```python
from build123d import *

# Parameters (mm, degrees)
SKETCH1_W           = 76.2
SKETCH1_H           = 76.2
BOSS_EXTRUDE1_DEPTH = 2.9718
SKETCH2_W           = 2.9718
SKETCH2_H           = 38.1
CUT_EXTRUDE1_DEPTH  = 54.963428313
CUT_EXTRUDE7_DEPTH  = 54.963428313
SKETCH8_W           = 1.7526
SKETCH8_H           = 2.38125
CUT_EXTRUDE8_DEPTH  = 54.963428313


with BuildPart() as part:
    # Sketch1 → Boss-Extrude1 (new body)
    with BuildSketch(Plane(origin=(0, 0, 0), x_dir=(1, 0, 0), z_dir=(0, 1, 0))):
        Rectangle(SKETCH1_W, SKETCH1_H)
    extrude(amount=BOSS_EXTRUDE1_DEPTH)

    # Sketch2 → Cut-Extrude1 (cut, through all)
    with BuildSketch(Plane(origin=(0, 2.9718, 0), x_dir=(1, 0, 0), z_dir=(0, 1, 0))):
        with Locations((36.6141, 0)):
            Rectangle(SKETCH2_W, SKETCH2_H)
    cut_extrude1 = extrude(amount=-CUT_EXTRUDE1_DEPTH, mode=Mode.SUBTRACT)

    # Sketch7 → Cut-Extrude7 (cut, through all)
    with BuildSketch(Plane(origin=(0, 2.9718, 0), x_dir=(1, 0, 0), z_dir=(0, 1, 0))):
        Polygon((35.1282, 1.4224), (29.05125, 1.4224), (29.05125, 3.175), (26.67, 3.175), (26.67, 1.4224), (22.86, 1.4224), (22.86, -1.4224), (26.67, -1.4224), (26.67, -3.175), (29.05125, -3.175), (29.05125, -1.4224), (35.1282, -1.4224), align=None)
    cut_extrude7 = extrude(amount=-CUT_EXTRUDE7_DEPTH, mode=Mode.SUBTRACT)

    # Sketch8 → Cut-Extrude8 (cut, through all)
    with BuildSketch(Plane(origin=(0, 2.9718, 0), x_dir=(1, 0, 0), z_dir=(0, 1, 0))):
        Polygon((25.4, 38.1), (-12.7, 38.1), (-12.7, 35.1282), (4.9276, 35.1282), (7.7724, 35.1282), (25.4, 35.1282), align=None)
        Polygon((7.7724, 35.1282), (4.9276, 35.1282), (4.9276, 29.05125), (4.9276, 26.67), (4.9276, 22.86), (7.7724, 22.86), (7.7724, 26.67), (7.7724, 29.05125), align=None)
        with Locations((8.6487, 27.860625)):
            Rectangle(SKETCH8_W, SKETCH8_H)
        with Locations((4.0513, 27.860625)):
            Rectangle(SKETCH8_W, SKETCH8_H)
    extrude(amount=-CUT_EXTRUDE8_DEPTH, mode=Mode.SUBTRACT)

    # Mirror1: Cut-Extrude1, Cut-Extrude7 across plane
    add(cut_extrude1.mirror(Plane(origin=(0, 0, 0), x_dir=(0, 0, 1), z_dir=(1, 0, 0))), mode=Mode.SUBTRACT)
    add(cut_extrude7.mirror(Plane(origin=(0, 0, 0), x_dir=(0, 0, 1), z_dir=(1, 0, 0))), mode=Mode.SUBTRACT)


solid = part.part
```
Design review of the part built by this model. Coordinates are the model's own, in mm. A direction names the side the tool comes from. Give positions to 0.01 mm unless a question says otherwise; leave off trailing zeros. Order: outer loops, then holes, each group sorted by start corner. A loop starts at its lowest first (then second) coordinate and runs counter-clockwise, first axis right, second up. Notation, with made-up numbers: M 87,-31 L 115,-31 A19 cw 115,-3 Z; hole C 67,5.5 d2. An arc over 180 degrees is marked long. One line per question, with ' | ' between items. Start each with the question number.
Q1. Machinability: for faces 4 (the face through (29.051, 2, 2)), 5 (the face through (7.772, 2, -32)), 6 (the face through (-25, 2, 1.422)), which of the approach directions +Z, -Z, +X, -X, +Y, -Y give a long, thin tool a straight path to every point of the face, cutting with its end or side? Answer none if there is none.
Q2. The part is to be moulded in two halves that separate along X. For faces 1 (the face through (-35.128, 2, 10)), 2 (the face through (32, 1, -38.1)), 3 (the face through (4, 2, -26.67)), say which applies: +X half, -X half, draft (parallel to the pull), parting line (faces both ways), or undercut.
Q3. For L1, parallel to Z at x = 28.5, y = 2.4 (3 decimals); L2, parallel to Z at x = 33.5, y = 2.6; L3, parallel to Z at x = -11.5, y = 1.2, list the stretches that pass through material, from the lowest coordinate up. Write a range as [from, to].
Q4. We need section A-A (z = -24). Write out the cut boundary in (x, y).
Q5. For pin 1 Ø4 at (x, z) = (-3.5, 5.5) entering from -Y; pin 2 Ø0.5 at (y, z) = (2, -2.5) entering from +X; pin 3 Ø0.5 at (x, y) = (4, 2) entering from -Z; pin 4 Ø0.9 at (y, z) = (1.5, -2) entering from -X, all flat-tipped, find the tip position at first contact; note any pin that passes through.
Q6. We need section C-C (z = -5.5). Write out the cut boundary in (x, y).
Q7. We need section B-B (x = -6.5). Write out the cut boundary in (y, z), plus the area to 3 significant figures.
Returned:
1) face 4: +Y, -Y | face 5: -Z, +Y, -Y | face 6: -X, +Y, -Y
2) face 1: -X half | face 2: draft | face 3: undercut
3) L1: [-38.1, -3.175], [3.175, 38.1] | L2: [-38.1, -1.42], [1.42, 38.1] | L3: [-35.13, 38.1]
4) outline: M -38.1,0 L 4.93,0 L 4.93,2.97 L -38.1,2.97 Z; M 7.77,0 L 38.1,0 L 38.1,2.97 L 7.77,2.97 Z
5) pin 1: y = 0 | pin 2: x = 35.13 | pin 3: z = -35.13 | pin 4: x = -35.13
6) outline: M -35.13,0 L 35.13,0 L 35.13,2.97 L -35.13,2.97 Z
7) outline: M 0,-35.13 L 2.97,-35.13 L 2.97,38.1 L 0,38.1 Z | area: 218 mm2
